Autodesk Inventor part; units mm, degrees
ref_plane "YZ Plane" through (0, 0, 0) normal (1, 0, 0) x (0, 1, 0)
ref_plane "XZ Plane" through (0, 0, 0) normal (0, 1, 0) x (-1, 0, 0)
ref_plane "XY Plane" through (0, 0, 0) normal (0, 0, 1) x (1, 0, 0)
sketch "Sketch2" plane through (0, 0, 0) normal (0, 1, 0) x (-1, 0, 0)
  line L0 (-10.25, 10.25) -> (10.25, 10.25)
  line L1 (10.25, 10.25) -> (10.25, -10.25)
  line L2 (10.25, -10.25) -> (-10.25, -10.25)
  line L3 (-10.25, -10.25) -> (-10.25, 10.25)
  line L4 (-10.25, 10.25) -> (10.25, -10.25) construction
  line L5 (10.25, 10.25) -> (-10.25, -10.25) construction
  line L6 (-15, 15) -> (15, 15)
  line L7 (15, 15) -> (15, -15)
  line L8 (15, -15) -> (-15, -15)
  line L9 (-15, -15) -> (-15, 15)
  line L10 (-15, 15) -> (15, -15) construction
  line L11 (15, 15) -> (-15, -15) construction
  point P0 (0, 0)
  dimension "d2" = 20.5
  dimension "d3" = 20.5
  dimension "d4" = 30
  dimension "d5" = 30
extrude "Extrusion1" add sketch "Sketch2" along normal blind 20
sketch "Sketch3" plane through (-10.25, 0, -10.25) normal (0, 0, 1) x (1, 0, 0)
  circle A0 centre (9.9, 16) radius 2.05
  circle A1 centre (4.7038, 7) radius 2.05
  circle A2 centre (15.0962, 7) radius 2.05
  point P0 (10.25, 0)
  point P1 (9.9, 10)
  dimension "d8" = 4.1
  dimension "d9" = 6
  dimension "d12" = 360
extrude "Extrusion2" cut sketch "Sketch3" along normal through all both and the other way through all
sketch "Sketch4" plane through (0, 0, 0) normal (0, -1, 0) x (1, 0, 0)
  line L0 (-15, -15) -> (15, -15)
  line L1 (15, -15) -> (15, 15)
  line L2 (15, 15) -> (-15, 15)
  line L3 (-15, 15) -> (-15, -15)
  line L4 (-15, -15) -> (15, 15) construction
  line L5 (15, -15) -> (-15, 15) construction
  point P0 (0, 0)
  dimension "d16" = 30
  dimension "d17" = 30
extrude "Extrusion3" add sketch "Sketch4" along normal blind 25
sketch "Sketch5" plane through (0, -25, 0) normal (0, -1, 0) x (1, 0, 0)
  circle A0 centre (0, 0) radius 20
  line L0 (-20, 0) -> (20, 0)
  dimension "d20" = 40
revolve "Revolution1" cut sketch "Sketch5" angle 360 about axis through (-20, -25, 0) along (1, 0, 0) picked at (4.9901, 4.4208) contours L0 A0
sketch "Sketch6" plane through (0, -25, 0) normal (0, -1, 0) x (1, 0, 0)
  line L0 (-22.5, 22.5) -> (22.5, 22.5)
  line L1 (22.5, 22.5) -> (22.5, -22.5)
  line L2 (22.5, -22.5) -> (-22.5, -22.5)
  line L3 (-22.5, -22.5) -> (-22.5, 22.5)
  line L4 (-22.5, 22.5) -> (22.5, -22.5) construction
  line L5 (22.5, 22.5) -> (-22.5, -22.5) construction
  point P0 (0, 0)
  dimension "d23" = 45
  dimension "d24" = 45
extrude "Extrusion4" cut sketch "Sketch6" against normal blind 15
fillet "Fillet2" radius 5.5 8 edges at (0, -10, 15) (15, -10, 0) (0, -10, -15) (-15, -10, 0) (15, 5, -15) (-15, 5, -15) (-15, 5, 15) (15, 5, 15)
equation "\"d2\" = tool_mount_side + clearance"
equation "\"d3\" = tool_mount_side + clearance"
equation "\"d6\" = tool_mount_depth"
equation "\"tool_mount_side\" = 20"
equation "\"clearance\" = 0.5"
equation "\"tool_mount_depth\" = 20"
properties part number "tool_shoe"
Part model, mm, in its own coordinate system. A direction names the side the tool comes from. Round coordinates to 2 decimals unless told otherwise and drop trailing zeros. Write each loop counter-clockwise with the first axis right and the second up, starting at its lowest first coordinate (ties: lowest second). Pieces come first, ordered by that corner, then holes.
Item 1: Probe L1, parallel to X at y = 3, z = -7.5; L2, parallel to X at y = 7, z = 13. List the from-to ranges inside material, lowest first.
Results:
L1: x = -15 to -10.25, 10.25 to 15
L2: x = -13.74 to -7.6, -3.5 to 2.8, 6.9 to 13.74
Item 2: Drop flat-ended pins along their axis: pin 1 Ø3 at (x, z) = (-2, -4) entering from +Y; pin 2 Ø3 at (x, z) = (11, 11.5) entering from -Y; pin 3 Ø1.5 at (x, z) = (8.5, 3) entering from -Y. Give the stop position or say it passes through.
Results:
pin 1: stops at y = 0
pin 2: stops at y = -9.91
pin 3: stops at y = -7.55
Item 3: Which spindle directions (+Z, -Z, +X, -X, +Y, -Y) get a long thin tool onto all of the face, cutting with end or side? Do faces 4 (the flat face through (10.25, 10, 0)), 5 (the flat face through (0, 8, 15)). Say none if no direction does.
Results:
face 4: +Y
face 5: +Z, +X, -X, +Y, -Y
Item 4: Cut at D-D, the plane z = -7. Give the cut face in (x, y) (3 decimals), plus the area to 3 significant figures.
Results:
outline: (-15, -4.5) arc R5.5 ccw to (-10.957, -9.803) arc R18.735 cw to (10.957, -9.803) arc R5.5 ccw to (15, -4.5) - (15, 20) - (10.25, 20) - (10.25, 0) - (-10.25, 0) - (-10.25, 20) - (-15, 20) - close
area: 420 mm2
Item 5: Two-plate mould, pull along X, no slides. Class faces 1 (the flat face through (-13, 20, 0)), 2 (the cylindrical face through (-13.35, 7.92, -13.43)), 3 (the flat face through (0, 10, -10.25)): +X half, -X half, draft (parallel to the pull), parting line (faces both ways), or undercut.
Results:
face 1: draft
face 2: -X half
face 3: undercut
Item 6: Cut at C-C, the plane x = -4. Give the cut face in (y, z).
Results:
outline: (-9.44, -11.91) arc R5.5 ccw to (-4.5, -15) - (5.65, -15) - (5.65, -10.25) - (0, -10.25) - (0, 10.25) - (5.65, 10.25) - (5.65, 15) - (-4.5, 15) arc R5.5 ccw to (-9.44, 11.91) arc R19.6 cw to start; (8.35, -15) - (20, -15) - (20, -10.25) - (8.35, -10.25) - close; (8.35, 10.25) - (20, 10.25) - (20, 15) - (8.35, 15) - close
Item 7: Cut at B-B, the plane y = 16. Give the cut face in (x, z), plus the area to 3 significant figures.
Results:
outline: (-15, -9.5) arc R5.5 ccw to (-9.5, -15) - (-2.4, -15) - (-2.4, -10.25) - (-10.25, -10.25) - (-10.25, 10.25) - (-2.4, 10.25) - (-2.4, 15) - (-9.5, 15) arc R5.5 ccw to (-15, 9.5) - close; (1.7, -15) - (9.5, -15) arc R5.5 ccw to (15, -9.5) - (15, 9.5) arc R5.5 ccw to (9.5, 15) - (1.7, 15) - (1.7, 10.25) - (10.25, 10.25) - (10.25, -10.25) - (1.7, -10.25) - close
area: 415 mm2
Item 8: Cut at A-A, the plane y = 7. Give the cut face in (x, z).
Results:
outline: (-15, -9.5) arc R5.5 ccw to (-9.5, -15) - (-7.6, -15) - (-7.6, -10.25) - (-10.25, -10.25) - (-10.25, 10.25) - (-7.6, 10.25) - (-7.6, 15) - (-9.5, 15) arc R5.5 ccw to (-15, 9.5) - close; (-3.5, -15) - (2.8, -15) - (2.8, -10.25) - (-3.5, -10.25) - close; (-3.5, 10.25) - (2.8, 10.25) - (2.8, 15) - (-3.5, 15) - close; (6.9, -15) - (9.5, -15) arc R5.5 ccw to (15, -9.5) - (15, 9.5) arc R5.5 ccw to (9.5, 15) - (6.9, 15) - (6.9, 10.25) - (10.25, 10.25) - (10.25, -10.25) - (6.9, -10.25) - close
